Here's the drawing with two shaded views (mm, measured from the low corner). I have some questions. Round coordinates to 2 decimals unless told otherwise and drop trailing zeros. Loops run counter-clockwise (first coordinate to the right, second up) from the corner with the lowest first, then second, coordinate; pieces in that order, holes last. Notation, with made-up numbers: M -38.5,-17 L -0.5,-17 A19 cw -0.5,12 Z; hole C 85.5,-37 d6. An arc over 180 degrees is marked long. Answer as CSV lines item,"result".
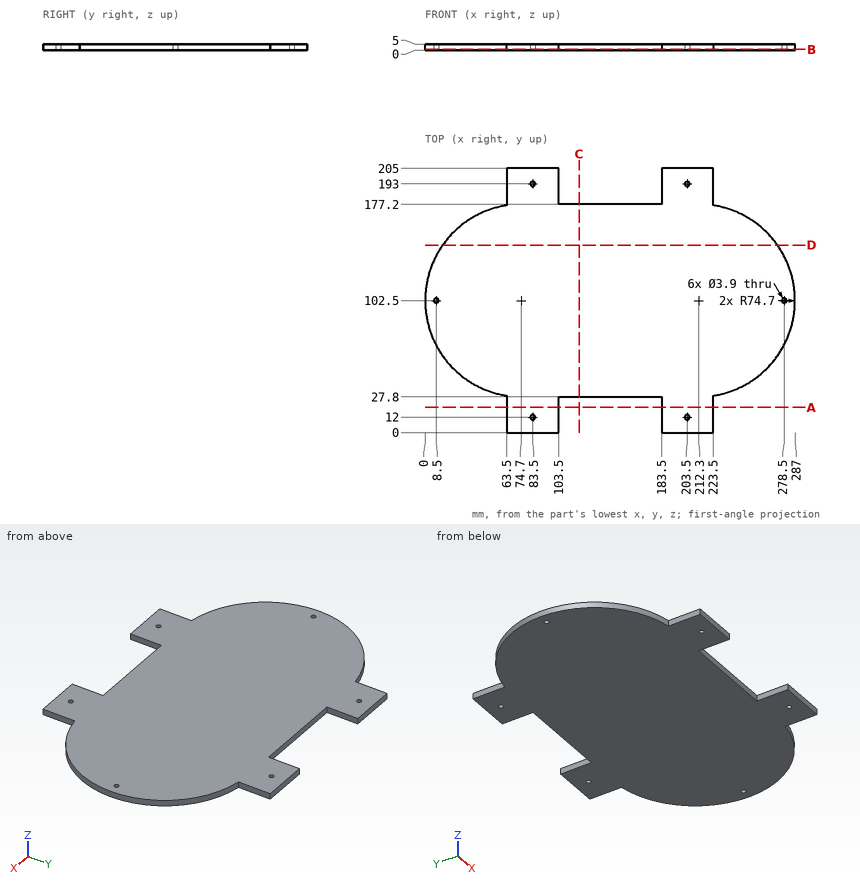
1. I want a section at A-A, the plane y = 19.5. Please give me the cut outline in (x, z).
Evaluation:
outline,"M 63.5,0 L 103.5,0 L 103.5,5 L 63.5,5 Z; M 183.5,0 L 223.5,0 L 223.5,5 L 183.5,5 Z"
2. For P1, Ø3, axis at x = 83.5, y = 193, coming from the +Z side; P2, Ø1, axis at y = 40, z = 3, coming from the +X side, each with a flat end and sliding along its axis, tell me the tip position at first contact or that it passes through.
Evaluation:
P1,"passes through"
P2,"stops at x = 253.97"
3. I want a section at D-D, the plane y = 145.5. Please give me the cut outline in (x, z).
Evaluation:
outline,"M 13.62,0 L 273.38,0 L 273.38,5 L 13.62,5 Z"
4. If I drill on line 1 (X direction, y = 193, z = 3.7); line 2 (X direction, y = 21.5, z = 1.25); line 3 (Y direction, x = 168, z = 4), over which ranges is the centre line in solid material (lowest first)? Write a range as [from, to].
Evaluation:
line 1,"x = [63.5, 81.55], [85.45, 103.5], [183.5, 201.55], [205.45, 223.5]"
line 2,"x = [63.5, 103.5], [183.5, 223.5]"
line 3,"y = [27.8, 177.2]"
5. I want a section at B-B, the plane z = 0.8. Please give me the cut outline in (x, y), and give its area (3 significant figures).
Evaluation:
outline,"M 63.5,0 L 103.5,0 L 103.5,27.8 L 183.5,27.8 L 183.5,0 L 223.5,0 L 223.5,28.64 A74.7 ccw 223.5,176.36 L 223.5,205 L 183.5,205 L 183.5,177.2 L 103.5,177.2 L 103.5,205 L 63.5,205 L 63.5,176.36 A74.7 ccw 63.5,28.64 Z; hole C 8.5,102.5 d3.9; hole C 83.5,12 d3.9; hole C 83.5,193 d3.9; hole C 203.5,12 d3.9; hole C 203.5,193 d3.9; hole C 278.5,102.5 d3.9"
area,"42,500 mm²"
6. I want a section at C-C, the plane x = 119.5. Please give me the cut outline in (y, z), and give its area (3 significant figures).
Evaluation:
outline,"M 27.8,0 L 177.2,0 L 177.2,5 L 27.8,5 Z"
area,"747 mm²"
